from build123d import *

# Parameters (mm, degrees)
F0_W     = 293.2697534561
F0_H     = 120.0150027871
F1_DEPTH = 12.7
F2_W     = 19.1973745823
F2_H     = 81.7032158375
F2_W_2   = 13.0126923323
F3_DEPTH = 13.97
F4_W     = 293.2697534561
F4_H     = 20.2290192246
F5_DEPTH = 12.7
F6_W     = 83.4743231535
F6_H     = 13.97
F7_DEPTH = 8.636


with BuildPart() as f1:
    # F0 (on Front) → F1 (new body)
    with BuildSketch(Plane.XZ):
        Rectangle(F0_W, F0_H)
    extrude(amount=F1_DEPTH)

    # F2 (on face) → F3 (join)
    with BuildSketch(Plane.XZ.offset(12.7)):
        Polygon((146.6348767281, 60.0075013936), (-146.6348767281, 60.0075013936), (-146.6348767281, 42.1536527574), (-133.6221843958, 42.1536527574), (127.4375021458, 42.1536527574), (146.6348767281, 42.1536527574), align=None)
        with Locations((137.0361894369, 1.3020448387)):
            Rectangle(F2_W, F2_H)
        with Locations((-140.1285305619, 1.3020448387)):
            Rectangle(F2_W_2, F2_H)
        Polygon((-133.6221843958, -39.5495630801), (-146.6348767281, -39.5495630801), (-146.6348767281, -60.0075013936), (146.6348767281, -60.0075013936), (146.6348767281, -39.5495630801), (127.4375021458, -39.5495630801), align=None)
    extrude(amount=F3_DEPTH)

    # F4 (on face) → F5 (join)
    with BuildSketch(Plane(origin=(0, 0, 0), x_dir=(-1, 0, 0), z_dir=(0, 1, 0))):
        with Locations((0, 36.5786291659)):
            Rectangle(F4_W, F4_H)
    extrude(amount=F5_DEPTH)

    # F6 (on face) → F7 (cut)
    with BuildSketch(Plane(origin=(0, 0, 42.1536527574), x_dir=(1, 0, 0), z_dir=(0, 0, -1))):
        with Locations((-8.9395232499, 19.685)):
            Rectangle(F6_W, F6_H)
    extrude(amount=-F7_DEPTH, mode=Mode.SUBTRACT)


solid = f1.part
Build history of the part. All positions in model axes, mm. A direction names the side the tool comes from. Round coordinates to 2 decimals unless told otherwise and drop trailing zeros. Loops run counter-clockwise (first coordinate to the right, second up) from the corner with the lowest first, then second, coordinate; pieces in that order, holes last. Notation, with made-up numbers: (-39.75, 44) -> (-5.75, 44) arc R4 cw to (-5.75, 49) -> close; hole circle Ø9 at (54, 89). An arc over 180 degrees is marked (long way). Use CSV: the item, a comma, the result in double quotes. Start each with the question number.
Q1. Saw through at B-B on y = -24. Give the cut face in (x, z), and give its area (3 significant figures).
Q2. Flat gauge pins, fed straight in: pin 1 Ø3 at (x, z) = (-111, 35) entering from -Y; pin 2 Ø10 at (x, y) = (-63, 6) entering from +Z; pin 3 Ø4 at (x, z) = (48.5, 54.5) entering from +Y. Where does each tip first touch, or does it go through?
Q3. Saw through at D-D on y = 4.5. Give the cut face in (x, z).
Q4. Saw through at C-C on x = 6.5. Give the cut face in (y, z), and give its area (3 significant figures).
Q5. Which spindle directions (+Z, -Z, +X, -X, +Y, -Y) get a long thin tool onto all of the face, cutting with end or side? Do faces 1 (the face through (-2, 0, -16)), 2 (the face through (-2, 0, 53)), 3 (the face through (-10, -20, 50.79)), 4 (the face through (10, -26.67, -40)). Say none if no direction does.
Q6. Saw through at A-A on z = -10. Give the cut face in (x, y).
Q7. Mould opens along Z. For faces 5 (the face through (2, -13, 60.008)), 6 (the face through (-50.677, -20, 46)), 7 (the face through (2, 12.7, 37)), 8 (the face through (127.438, -20, 1)) say: +Z half, -Z half, draft (parallel to the pull), parting line (faces both ways), or undercut.
Q8. Drill centre lines: L1, parallel to X at y = -22.5, z = 40.5; L2, parallel to Z at x = -27, y = -18; L3, parallel to Y at x = -43, z = 11.5. Where is each one in solid material? Low to high.
Solutions:
1,outline,"(-146.63, -60.01) -> (146.63, -60.01) -> (146.63, 60.01) -> (-146.63, 60.01) -> close; hole (-133.62, -39.55) -> (127.44, -39.55) -> (127.44, 42.15) -> (32.8, 42.15) -> (32.8, 50.79) -> (-50.68, 50.79) -> (-50.68, 42.15) -> (-133.62, 42.15) -> close"
1,area,"13,100 mm^2"
2,pin 1,"stops at y = -12.7"
2,pin 2,"stops at z = 46.69"
2,pin 3,"stops at y = 0"
3,outline,"(-146.63, 26.46) -> (146.63, 26.46) -> (146.63, 46.69) -> (-146.63, 46.69) -> close"
4,outline,"(-26.67, -60.01) -> (0, -60.01) -> (0, 26.46) -> (12.7, 26.46) -> (12.7, 46.69) -> (0, 46.69) -> (0, 60.01) -> (-26.67, 60.01) -> (-26.67, 50.79) -> (-12.7, 50.79) -> (-12.7, -39.55) -> (-26.67, -39.55) -> close"
4,area,"2,200 mm^2"
5,face 1,"-Z, +X, -X, +Y"
5,face 2,"+Z, +X, -X, +Y"
5,face 3,"-Y"
5,face 4,"+Z, -Z, +X, -X, -Y"
6,outline,"(-146.63, -26.67) -> (-133.62, -26.67) -> (-133.62, -12.7) -> (127.44, -12.7) -> (127.44, -26.67) -> (146.63, -26.67) -> (146.63, 0) -> (-146.63, 0) -> close"
7,face 5,"+Z half"
7,face 6,"undercut"
7,face 7,"draft"
7,face 8,"undercut"
8,L1,"x = -146.63 to -133.62, 127.44 to 146.63"
8,L2,"z = -60.01 to -39.55, 50.79 to 60.01"
8,L3,"y = -12.7 to 0"
